Autodesk Inventor part; units mm, degrees
ref_plane "YZ Plane" through (0, 0, 0) normal (1, 0, 0) x (0, 1, 0)
ref_plane "XZ Plane" through (0, 0, 0) normal (0, 1, 0) x (-1, 0, 0)
ref_plane "XY Plane" through (0, 0, 0) normal (0, 0, 1) x (1, 0, 0)
sketch "スケッチ1" plane through (0, 0, 0) normal (0, 0, 1) x (1, 0, 0)
  circle A0 centre (0, 0) radius 12.5
  line L0 (-1.35, 12.5) -> (1.35, 12.5) construction
  line L1 (1.35, 12.5) -> (1.35, 9.8)
  line L2 (1.35, 9.8) -> (-1.35, 9.8)
  line L3 (-1.35, 9.8) -> (-1.35, 12.5)
  line L4 (-5.4684, 8.2438) -> (-6.6399, 10.6764)
  line L5 (-4.2072, 11.8479) -> (-3.0358, 9.4152)
  line L6 (-3.0358, 9.4152) -> (-5.4684, 8.2438)
  line L7 (-8.5037, 5.0547) -> (-10.6146, 6.7382)
  line L8 (-8.9312, 8.8491) -> (-6.8202, 7.1657)
  line L9 (-6.8202, 7.1657) -> (-8.5037, 5.0547)
  line L10 (-9.8547, 0.8646) -> (-12.487, 1.4654)
  line L11 (-11.8862, 4.0977) -> (-9.2539, 3.4969)
  line L12 (-9.2539, 3.4969) -> (-9.8547, 0.8646)
  line L13 (-9.2539, -3.4969) -> (-11.8862, -4.0977)
  line L14 (-12.487, -1.4654) -> (-9.8547, -0.8646)
  line L15 (-9.8547, -0.8646) -> (-9.2539, -3.4969)
  line L16 (-6.8202, -7.1657) -> (-8.9312, -8.8491)
  line L17 (-10.6146, -6.7382) -> (-8.5037, -5.0547)
  line L18 (-8.5037, -5.0547) -> (-6.8202, -7.1657)
  line L19 (-3.0358, -9.4152) -> (-4.2072, -11.8479)
  line L20 (-6.6399, -10.6764) -> (-5.4684, -8.2438)
  line L21 (-5.4684, -8.2438) -> (-3.0358, -9.4152)
  line L22 (1.35, -9.8) -> (1.35, -12.5)
  line L23 (-1.35, -12.5) -> (-1.35, -9.8)
  line L24 (-1.35, -9.8) -> (1.35, -9.8)
  line L25 (5.4684, -8.2438) -> (6.6399, -10.6764)
  line L26 (4.2072, -11.8479) -> (3.0358, -9.4152)
  line L27 (3.0358, -9.4152) -> (5.4684, -8.2438)
  line L28 (8.5037, -5.0547) -> (10.6146, -6.7382)
  line L29 (8.9312, -8.8491) -> (6.8202, -7.1657)
  line L30 (6.8202, -7.1657) -> (8.5037, -5.0547)
  line L31 (9.8547, -0.8646) -> (12.487, -1.4654)
  line L32 (11.8862, -4.0977) -> (9.2539, -3.4969)
  line L33 (9.2539, -3.4969) -> (9.8547, -0.8646)
  line L34 (9.2539, 3.4969) -> (11.8862, 4.0977)
  line L35 (12.487, 1.4654) -> (9.8547, 0.8646)
  line L36 (9.8547, 0.8646) -> (9.2539, 3.4969)
  line L37 (6.8202, 7.1657) -> (8.9312, 8.8491)
  line L38 (10.6146, 6.7382) -> (8.5037, 5.0547)
  line L39 (8.5037, 5.0547) -> (6.8202, 7.1657)
  line L40 (3.0358, 9.4152) -> (4.2072, 11.8479)
  line L41 (6.6399, 10.6764) -> (5.4684, 8.2438)
  line L42 (5.4684, 8.2438) -> (3.0358, 9.4152)
  point P0 (0, 12.5)
  point P1 (-1.35, 12.4269)
  point P2 (-4.1755, 11.782)
  point P3 (-6.6081, 10.6105)
  point P4 (-8.874, 8.8035)
  point P5 (-10.5574, 6.6926)
  point P6 (-11.8149, 4.0814)
  point P7 (-12.4157, 1.4491)
  point P8 (-12.4157, -1.4491)
  point P9 (-11.8149, -4.0814)
  point P10 (-10.5574, -6.6926)
  point P11 (-8.874, -8.8035)
  point P12 (-6.6081, -10.6105)
  point P13 (-4.1755, -11.782)
  point P14 (-1.35, -12.4269)
  point P15 (1.35, -12.4269)
  point P16 (4.1755, -11.782)
  point P17 (6.6081, -10.6105)
  point P18 (8.874, -8.8035)
  point P19 (10.5574, -6.6926)
  point P20 (11.8149, -4.0814)
  point P21 (12.4157, -1.4491)
  point P22 (12.4157, 1.4491)
  point P23 (11.8149, 4.0814)
  point P24 (1.35, 12.4269)
  point P25 (10.5574, 6.6926)
  point P26 (8.874, 8.8035)
  point P27 (6.6081, 10.6105)
  point P28 (4.1755, 11.782)
  dimension "d0" = 25
  dimension "d3" = 2.7
  dimension "d4" = 2.7
  dimension "d7" = 360
extrude "押し出し2" add sketch "スケッチ1" along normal blind 2.5 contours A0 L31 L33 L32 L28 L30 L29 L25 L27 L26 L22 L24 L23 L19 L21 L20 L16 L18 L17 L13 L15 L14 L10 L12 L11 L7 L9 L8 L4 L6 L5 L3 L2 L1 L40 L42 L41 L37 L39 L38 L34 L36 L35
sketch "スケッチ2" plane through (-1.35, 9.8, 0) normal (1, 0, 0) x (0, 0, -1)
  line L0 (0, 0) -> (0, 2.6269)
  circle A0 centre (0, 2.6269) radius 1.1
  point P0 (0, -9.8)
  dimension "d11" = 2.2
extrude "押し出し3" cut sketch "スケッチ2" against normal blind 1
properties part number "frame"
Read the model definition and answer for the solid it produces. Units are mm, in the model's axes. A direction names the side the tool comes from. Give positions to 0.01 mm unless a question says otherwise; leave off trailing zeros. Write each loop counter-clockwise with the first axis right and the second up, starting at its lowest first coordinate (ties: lowest second). Pieces come first, ordered by that corner, then holes. Notation, with made-up numbers: M -23.5,-5.75 L 8.5,-5.75 A32 ccw 8.5,25.25 Z; hole C 3.25,30.5 d5. An arc over 180 degrees is marked long. Put each result on its own line as item: value. Start each with the question number.
1. For a pull along X with two mould halves and no side action, classify faces 5 (the flat face through (-3.598, -10.582, 1.232)), 6 (the flat face through (-4.27, -8.82, 1.23)), 7 (the cylindrical face through (2.801, -12.182, 1.232)), 8 (the cylindrical face through (-11.253, -5.442, 1.232)) as released by +X, released by -X, zero draft, split by the parting line, or undercut.
2. Consider line 1 along Y through (x, z) = (-11, 0.4); line 2 along Y through (x, z) = (4, 0.9); line 3 along X through (y, z) = (-11, 2). Determine where each line is inside the solid, lowest interval first.
3. The part is cut by section C-C, the plane x = -1. Give the vertices of the cut face in (y, z), and give its area (3 significant figures).
4. Which of the six approach directions +Z, -Z, +X, -X, +Y, -Y give full straight-line access (tool end or side, diameter ignored) to faces 1 (the flat face through (1.35, 11, 1)), 2 (the flat face through (-11.117, 1.153, 1.232)), 3 (the flat face through (-10.516, -3.785, 1.232)), 4 (the flat face through (-2.35, 11.9, 0.4))?
5. The part is cut by section D-D, the plane y = 2.25. Give the vertices of the cut face in (x, z), and give its area (3 significant figures).
6. The part is cut by section A-A, the plane x = -3.5. Give the vertices of the cut face in (y, z).
7. The part is cut by section B-B, the plane y = -6. Give the vertices of the cut face in (x, z), and give its area (3 significant figures).
8. Each of these flat-tipped pins is pushed along its axis until it touches: pin 1 Ø1 at (x, z) = (2.5, 2) entering from +Y; pin 2 Ø1 at (x, z) = (-4, 1) entering from +Y; pin 3 Ø6 at (x, y) = (1.5, -1) entering from -Z; pin 4 Ø1 at (y, z) = (12, 0.5) entering from +X. Where does it stop, or does it pass through?
Final values:
1. face 5: undercut
1. face 6: undercut
1. face 7: released by +X
1. face 8: released by -X
2. line 1: y = -5.94 to -3.9, -1.13 to 1.13, 3.9 to 5.94
2. line 2: y = -11.84 to -11.42, -8.95 to 8.95, 11.42 to 11.84
2. line 3: x = -3.8 to -1.35, 1.35 to 3.8
3. outline: M -9.8,0 L 9.8,0 L 9.8,2.5 L -9.8,2.5 Z
3. area: 49.0 mm²
4. face 1: +Z, -Z, +Y
4. face 2: +Z, -Z
4. face 3: +Z, -Z, -X
4. face 4: -Z, +Y
5. outline: M -9.54,0 L 9.54,0 L 9.54,2.5 L -9.54,2.5 Z
5. area: 47.7 mm²
6. outline: M -12,0 L -10.38,0 L -10.38,2.5 L -12,2.5 Z; M -9.19,0 L 9.19,0 L 9.19,2.5 L -9.19,2.5 Z; M 10.38,0 L 12,0 L 12,2.5 L 10.38,2.5 Z
7. outline: M -10.97,0 L -9.69,0 L -9.69,2.5 L -10.97,2.5 Z; M -7.75,0 L 7.75,0 L 7.75,2.5 L -7.75,2.5 Z; M 9.69,0 L 10.97,0 L 10.97,2.5 L 9.69,2.5 Z
7. area: 45.1 mm²
8. pin 1: stops at y = 12.34
8. pin 2: stops at y = 12
8. pin 3: stops at z = 0
8. pin 4: stops at x = 4.18
